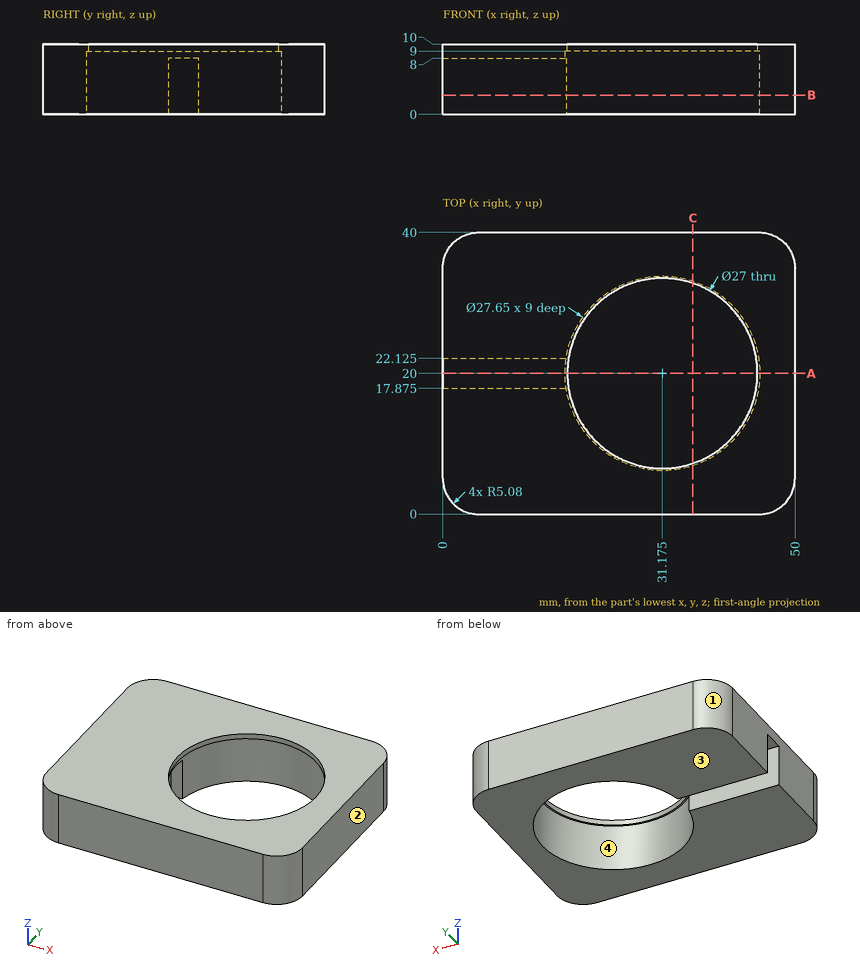
Check sheet for the drawn part. Datum: minimum x, y, z corner. Units: mm. Round coordinates to 2 decimals unless told otherwise and drop trailing zeros. Loops run counter-clockwise (first coordinate to the right, second up) from the corner with the lowest first, then second, coordinate; pieces in that order, holes last. Notation, with made-up numbers: (-3.75, 59) - (15.25, 59) arc R27 cw to (15.25, 96) - close; hole circle Ø3 at (73, 28.25). An arc over 180 degrees is marked (long way). Answer as a JSON object with one key per item and string values. Group by question number.
Q1. Gauge pin test, flat ends, axial feed: P1, Ø21.5, axis at x = 31.175, y = 20, coming from the +Z side; P2, Ø2, axis at x = 9, y = 19.5, coming from the -Z side. Record the tip position at first contact, or that the pin passes through.
Q2. Sectioned sample at C-C, the plane x = 35.5. Enter the section's corners in (y, z).
Q3. Mould release check, pull along X, two halves, no side actions. Record for the marked faces 1, 2, 3 and 4: released by +X, released by -X, zero draft, split by the parting line, or undercut.
Q4. Sectioned sample at A-A, the plane y = 20. Enter the section's corners in (x, z) (3 decimals).
Q5. Scan lines: line 1 along Y through (x, z) = (15.5, 7.25) (3 decimals); line 2 along Z through (x, y) = (18, 16); line 3 along Y through (x, z) = (24, 7.5). Record each from-to range of solid material in increasing order. Write a range as [from, to].
Q6. Sectioned sample at B-B, the plane z = 2.75. Enter the section's corners in (x, y) (3 decimals), plus the area to 3 significant figures.
Solution:
{
 "1": {"P1": "passes through", "P2": "stops at z = 8"},
 "2": {"outline": "(0, 0) - (6.87, 0) - (6.87, 9) - (7.21, 9) - (7.21, 10) - (0, 10) - close; (32.79, 9) - (33.13, 9) - (33.13, 0) - (40, 0) - (40, 10) - (32.79, 10) - close"},
 "3": {"face 1": "released by -X", "face 2": "released by +X", "face 3": "zero draft", "face 4": "undercut"},
 "4": {"outline": "(0, 8) - (17.35, 8) - (17.35, 9) - (17.675, 9) - (17.675, 10) - (0, 10) - close; (44.675, 9) - (45, 9) - (45, 0) - (50, 0) - (50, 10) - (44.675, 10) - close"},
 "5": {"line 1": "y = [0, 17.875], [22.125, 40]", "line 2": "z = [9, 10]", "line 3": "y = [0, 8.18], [31.82, 40]"},
 "6": {"outline": "(0, 5.08) arc R5.08 ccw to (5.08, 0) - (44.92, 0) arc R5.08 ccw to (50, 5.08) - (50, 34.92) arc R5.08 ccw to (44.92, 40) - (5.08, 40) arc R5.08 ccw to (0, 34.92) - (0, 22.125) - (17.514, 22.125) arc R13.825 cw (long way) to (17.514, 17.875) - (0, 17.875) - close", "area": "1,300 mm²"}
}
